For this review, take the finished solid that the model builds, in its own axes (mm). A direction names the side the tool comes from. Give positions to 0.01 mm unless a question says otherwise; leave off trailing zeros. Order: outer loops, then holes, each group sorted by start corner. A loop starts at its lowest first (then second) coordinate and runs counter-clockwise, first axis right, second up. Notation, with made-up numbers: (-34, 11) - (18, 11) arc R13 cw to (18, 17) - close; hole circle Ø4 at (34, 15.5). An arc over 180 degrees is marked (long way). Use a Markdown table: item, result. Add a question column.
1) Clearance check with flat-ended pins moving along their axes: P1, Ø1.3, axis at x = 0, y = 1, coming from the +Z side; P2, Ø1, axis at x = -2, z = 25.5, coming from the -Y side; P3, Ø2, axis at x = 2, z = 18, coming from the +Y side; P4, Ø1.9, axis at x = -1.5, y = 0, coming from the -Z side. State where each tip first meets the part, or that it passes through.
2) Wall thickness on L1, parallel to Z at x = -1.25, y = 1.25 (3 decimals); L2, parallel to Z at x = 3, y = 0.75; L3, parallel to X at y = -0.75, z = 19: over which ranges is each line inside the solid? List them lowest first.
3) Machinability: for faces 1 (the face through (-0.34, -1.55, 30.14)), 2 (the face through (0, 0, 33.338)), 3 (the face through (3.03, 0.95, 32.92)), 4 (the face through (2, 0, 25.4)), which of the approach directions +Z, -Z, +X, -X, +Y, -Y give a long, thin tool a straight path to every point of the face, cutting with its end or side? Answer none if there is none.
4) Mouldability with a two-part tool opening along X and no side actions: class faces 5 (the face through (-0.794, 0, 34)), 6 (the face through (0.794, 0, 34)), 7 (the face through (0, 0, 0)), 8 (the face through (-0.34, -1.55, 12.52)) as released by +X, released by -X, zero draft, split by the parting line, or undercut.
5) We need section B-B on z = 20. Write out the cut boundary in (x, y) (1 decimal), then the cut area to 3 significant figures.
```python
from build123d import *

# Parameters (mm, degrees)
F0_R     = 1.5875
F1_DEPTH = 25.4
F2_R     = 3.175
F3_DEPTH = 3.175
F4_R     = 1.5875
F5_DEPTH = 3.175
F6_R     = 3.175
F7_DEPTH = 3.175
F8_W     = 1.5875
F8_H     = 6.35
F9_DEPTH = 1.5875
F10_SIZE = 0.79375


with BuildPart() as f1:
    # F0 (on Top) → F1 (new body)
    with BuildSketch(Plane.XY):
        Circle(F0_R)
    extrude(amount=F1_DEPTH)

    # F2 (on face) → F3 (join)
    with BuildSketch(Plane.XY.offset(25.4)):
        Circle(F2_R)
    extrude(amount=F3_DEPTH)

    # F4 (on face) → F5 (join)
    with BuildSketch(Plane.XY.offset(28.575)):
        Circle(F4_R)
    extrude(amount=F5_DEPTH)

    # F6 (on face) → F7 (join)
    with BuildSketch(Plane.XY.offset(31.75)):
        Circle(F6_R)
    extrude(amount=F7_DEPTH)

    # F8 (on face) → F9 (cut)
    with BuildSketch(Plane.XY.offset(34.925)):
        Rectangle(F8_W, F8_H)
    extrude(amount=-F9_DEPTH, mode=Mode.SUBTRACT)

    # F10
    f10_edges = [f1.edges().sort_by_distance(p)[0] for p in [
        (-3.175, 0, 34.925),
        (2.510058, 1.944282, 34.925),
        (2.510058, -1.944282, 34.925),
        (-3.175, 0, 28.575),
        (-3.175, 0, 25.4),
    ]]
    chamfer(f10_edges, length=F10_SIZE)


solid = f1.part
```
Checked values:
| question | item | result |
|---|---|---|
| 1 | P1 | z = 33.34 |
| 1 | P2 | y = -2.33 |
| 1 | P3 | y = 1.23 |
| 1 | P4 | z = 0 |
| 2 | L1 | 25.4 to 28.575, 31.75 to 34.925 |
| 2 | L2 | 26.11 to 27.86, 31.75 to 34.21 |
| 2 | L3 | -1.4 to 1.4 |
| 3 | face 1 | none |
| 3 | face 2 | +Z, +Y, -Y |
| 3 | face 3 | +Z, -Z |
| 3 | face 4 | -Z |
| 4 | face 5 | undercut |
| 4 | face 6 | undercut |
| 4 | face 7 | zero draft |
| 4 | face 8 | split by the parting line |
| 5 | outline | circle Ø3.2 at (0, 0) |
| 5 | area | 7.92 mm² |
